The model under review builds one solid part; all positions refer to its coordinate system, in mm. A direction names the side the tool comes from. Round coordinates to 2 decimals unless told otherwise and drop trailing zeros. Write each loop counter-clockwise with the first axis right and the second up, starting at its lowest first coordinate (ties: lowest second). Pieces come first, ordered by that corner, then holes. Notation, with made-up numbers: (10.5, -11) -> (33.5, -11) arc R17 cw to (33.5, 0) -> close; hole circle Ø10 at (-12.5, 57). An arc over 180 degrees is marked (long way). Answer as a JSON object with one key per item and string values. Group by question number.
1) We need section C-C, the plane y = 0. Write out the cut boundary in (x, z).
2) Machinability: for faces 4 (the cylindrical face through (-0.582, 28.694, -5.916)), 5 (the flat face through (0, 29, -12)), which of the approach directions +Z, -Z, +X, -X, +Y, -Y give a long, thin tool a straight path to every point of the face, cutting with its end or side? Answer none if there is none.
3) To check wall thickness, follow probe 1 along Y at (x, z) = (0, 0.65); probe 2 along Y at (x, z) = (0, -4.25); probe 3 along Z at (x, y) = (6.5, 14). State the ranges of each line that lie inside material, in increasing order. Write a range as [from, to].
4) Insertion check: pin 1 Ø5 at (x, y) = (-11.5, 17) entering from -Z; pin 2 Ø4 at (x, z) = (-13, -2.5) entering from -Y; pin 3 Ø1 at (x, z) = (19, -4.5) entering from -Y; pin 4 Ø3 at (x, y) = (0, 0) entering from +Z. Each pin has a flat end and moves straight along its axis. Give the tip position at first contact, or say it passes through.
5) We need section B-B, the plane x = 0. Write out the cut boundary in (y, z).
6) We need section D-D, the plane x = 20.5. Write out the cut boundary in (y, z), then the cut area to 3 significant figures.
7) Mouldability with a two-part tool opening along Y and no side actions: class faces 1 (the cylindrical face through (28.14, -8.86, -5.46)), 2 (the flat face through (0, 6, 0)), 3 (the flat face through (0, -6, 0.9)) as pulls with the +Y half, pulls with the -Y half, needs draft (parallel to the pull), parting line crosses it, or undercut.
from build123d import *

# Parameters (mm, degrees)
F0_R     = 29.5
F0_R_2   = 1.75
F1_DEPTH = 0.9
F2_R     = 29.5
F2_R_2   = 28.7
F3_DEPTH = 12
F4_W     = 59
F4_H     = 7
F5_DEPTH = 12


with BuildPart() as f1:
    # F0 (on Top) → F1 (new body)
    with BuildSketch(Plane.XY):
        Circle(F0_R)
        Circle(F0_R_2, mode=Mode.SUBTRACT)
    extrude(amount=F1_DEPTH)

    # F2 (on face) → F3 (join)
    with BuildSketch(Plane(origin=(0, 0, 0), x_dir=(1, 0, 0), z_dir=(0, 0, -1))):
        Circle(F2_R)
        Circle(F2_R_2, mode=Mode.SUBTRACT)
    extrude(amount=F3_DEPTH)

    # F4 (on face) → F5 (cut, through all)
    with BuildSketch(Plane(origin=(0, 0, -12), x_dir=(1, 0, 0), z_dir=(0, 0, -1))):
        Rectangle(F4_W, F4_H)
    extrude(amount=-F5_DEPTH, mode=Mode.SUBTRACT)


solid = f1.part
Here are the results:
{
 "1": {"outline": "(-29.5, 0) -> (-1.75, 0) -> (-1.75, 0.9) -> (-29.5, 0.9) -> close; (1.75, 0) -> (29.5, 0) -> (29.5, 0.9) -> (1.75, 0.9) -> close"},
 "2": {"face 4": "-Z", "face 5": "-Z, +X, -X, +Y, -Y"},
 "3": {"probe 1": "y = [-29.5, -1.75], [1.75, 29.5]", "probe 2": "y = [-29.5, -28.7], [28.7, 29.5]", "probe 3": "z = [0, 0.9]"},
 "4": {"pin 1": "stops at z = 0", "pin 2": "stops at y = -27.37", "pin 3": "stops at y = -22.98", "pin 4": "passes through"},
 "5": {"outline": "(-29.5, -12) -> (-28.7, -12) -> (-28.7, 0) -> (-1.75, 0) -> (-1.75, 0.9) -> (-29.5, 0.9) -> close; (1.75, 0) -> (28.7, 0) -> (28.7, -12) -> (29.5, -12) -> (29.5, 0.9) -> (1.75, 0.9) -> close"},
 "6": {"outline": "(-21.21, -12) -> (-20.09, -12) -> (-20.09, 0) -> (20.09, 0) -> (20.09, -12) -> (21.21, -12) -> (21.21, 0.9) -> (-21.21, 0.9) -> close", "area": "65.2 mm^2"},
 "7": {"face 1": "parting line crosses it", "face 2": "undercut", "face 3": "needs draft"}
}
